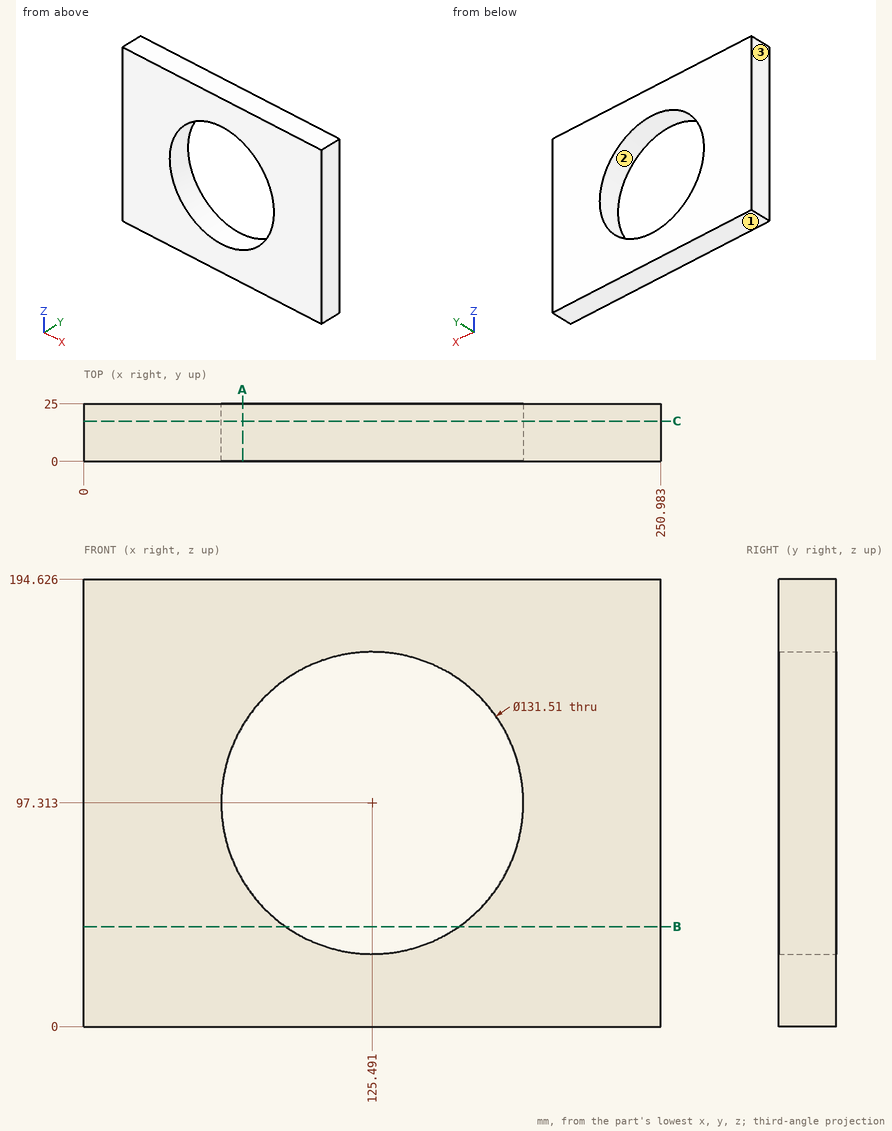
Here's the drawing with two shaded views (mm, measured from the low corner). I have some questions. Coordinates: 2 decimals unless noted, no trailing zeros. Order: outer loops, then holes, each group sorted by start corner. A loop starts at its lowest first (then second) coordinate and runs counter-clockwise, first axis right, second up.
Q1. Please list where these lines run through material, in increasing order: L1, parallel to Z at x = 107.5, y = 8 (1 decimal); L2, parallel to X at y = 5, z = 132.5 (1 decimal); L3, parallel to X at y = 1.75, z = 84 (1 decimal).
Q2. Thinking about a two-plate mould opening in Z: for the marked faces 1, 2 and 3, which applies, released by +Z, released by -Z, zero draft, split by the parting line, or undercut?
Q3. Suppose I cut it at C-C on y = 17.5. Please give me the cut outline in (x, z) (1 decimal).
Q4. Suppose I cut it at B-B on z = 43.5. Please give me the cut outline in (x, y) (1 decimal).
Q5. Suppose I cut it at A-A on x = 69. Please give me the cut outline in (y, z) (1 decimal), and give its area (3 significant figures).
Answer:
1. L1: z = 0 to 34.1, 160.6 to 194.6
1. L2: x = 0 to 69.9, 181 to 251
1. L3: x = 0 to 61.1, 189.9 to 251
2. face 1: released by -Z
2. face 2: undercut
2. face 3: zero draft
3. outline: (0, 0) - (251, 0) - (251, 194.6) - (0, 194.6) - close; hole circle Ø131.5 at (125.5, 97.3)
4. outline: (0, 0) - (87.7, 0) - (87.7, 25) - (0, 25) - close; (163.3, 0) - (251, 0) - (251, 25) - (163.3, 25) - close
5. outline: (0, 0) - (25, 0) - (25, 63.7) - (0, 63.7) - close; (0, 131) - (25, 131) - (25, 194.6) - (0, 194.6) - close
5. area: 3,180 mm2
